```python
from build123d import *

# Parameters (mm, degrees)
F0_W     = 66.9
F0_H     = 51.6
F1_DEPTH = 1.5
F2_R     = 33.44999
F3_R     = 1.625
F4_DEPTH = 1.5
F5_W     = 5.2
F5_H     = 3.85
F5_W_2   = 5.05
F6_DEPTH = 1.7


# Not quite as in the source:
# - a fillet or chamfer is up to 0.001 mm smaller than in the source, because OpenCascade refuses the exact size


with BuildPart() as f1:
    # F0 (on Top) → F1 (new body)
    with BuildSketch(Plane.XY):
        Rectangle(F0_W, F0_H)
    extrude(amount=F1_DEPTH)

    # F2 (radius 33.45 in the source; OpenCascade refuses exactly that, so slightly less here)
    f2_edges = [f1.edges().sort_by_distance(p)[0] for p in [
        (-33.45, 25.8, 0.75),
        (33.45, 25.8, 0.75),
    ]]
    fillet(f2_edges, radius=F2_R)

    # F3 (on Top) → F4 (cut)
    with BuildSketch(Plane.XY):
        with Locations((-21.525, 14.0641658831)):
            Circle(F3_R)
        with Locations((-14.025, 12.9547324661)):
            Circle(F3_R)
        with Locations((21.525, 14.0641658831)):
            Circle(F3_R)
        with Locations((14.025, 12.9547324661)):
            Circle(F3_R)
        with Locations((-29.5, -14.475)):
            Circle(F3_R)
        with Locations((29.5, -14.475)):
            Circle(F3_R)
    extrude(amount=F4_DEPTH, mode=Mode.SUBTRACT)

    # F5 (on face) → F6 (join)
    with BuildSketch(Plane.XY.offset(1.5)):
        with Locations((0, -7.525)):
            Rectangle(F5_W, F5_H)
        with Locations((0.075, 12.975)):
            Rectangle(F5_W_2, F5_H)
    extrude(amount=F6_DEPTH)


solid = f1.part
```
Verification items for the finished model (mm, model axes). A direction names the side the tool comes from. Coordinates: 2 decimals unless noted, no trailing zeros. Write each loop counter-clockwise with the first axis right and the second up, starting at its lowest first coordinate (ties: lowest second). Pieces come first, ordered by that corner, then holes. Notation, with made-up numbers: (62.5, 29) - (117.5, 29) arc R18 ccw to (117.5, 37) - close; hole circle Ø2 at (-24, 31.5). An arc over 180 degrees is marked (long way). Write item = value, one per line.
Q1. Access from +Z, -Z, +X, -X, +Y, -Y to the whole of each face (thin tool, end or side, straight path). Record for faces 1 (the face through (0, -5.6, 2)), 2 (the face through (-2.45, 13, 2)), 3 (the face through (2.6, -8, 2)), 4 (the face through (21.17, 12.48, 0.74)), 5 (the face through (0, 14.9, 2)).
Answer:
face_1 = +Z, +X, -X
face_2 = +Z, -X, +Y
face_3 = +Z, +X, +Y, -Y
face_4 = +Z, -Z
face_5 = +Z, +X, -X, +Y
Q2. Cross-section at C-C (x = -17.5). Enter the section's corners in (y, z).
Answer:
outline = (-25.8, 0) - (20.86, 0) - (20.86, 1.5) - (-25.8, 1.5) - close
Q3. Cross-section at A-A (z = 2.25). Enter the section's corners in (x, y), plus the area to 3 significant figures.
Answer:
outline = (-2.6, -9.45) - (2.6, -9.45) - (2.6, -5.6) - (-2.6, -5.6) - close; (-2.45, 11.05) - (2.6, 11.05) - (2.6, 14.9) - (-2.45, 14.9) - close
area = 39.5 mm²
Q4. Material ranges on L1, parallel to Y at x = 0, z = 1.85; L2, parallel to X at y = 11.5, z = 1.85; L3, parallel to Z at x = -13.5, y = -4, recorded low to high. Write a range as from..to.
Answer:
L1 = -9.45..-5.6, 11.05..14.9
L2 = -2.45..2.6
L3 = 0..1.5
Q5. Cross-section at B-B (x = -29.5). Enter the section's corners in (y, z), plus the area to 3 significant figures.
Answer:
outline = (-25.8, 0) - (-16.1, 0) - (-16.1, 1.5) - (-25.8, 1.5) - close; (-12.85, 0) - (8.12, 0) - (8.12, 1.5) - (-12.85, 1.5) - close
area = 46.0 mm²
Q6. Mould release check, pull along Z, two halves, no side actions. Record for faces 6 (the face through (12.735, 11.966, 0.74)), 7 (the face through (0, -5, 0)), 8 (the face through (0, -7, 3.2)): released by +Z, released by -Z, zero draft, split by the parting line, or undercut.
Answer:
face_6 = zero draft
face_7 = released by -Z
face_8 = released by +Z
Q7. Go/stop test with flat-tipped pins: pin 1 Ø3.5 at (x, y) = (14.02, 12.95) entering from +Z; pin 2 Ø2.5 at (x, y) = (-21.52, 14.06) entering from -Z; pin 3 Ø1.9 at (x, z) = (1, 2.5) entering from -Y; pin 4 Ø1.9 at (y, z) = (-6.5, 2) entering from -X. Record where each tip stops, or that it passes through.
Answer:
pin_1 = 1.5
pin_2 = through
pin_3 = -9.45
pin_4 = -33.45
Q8. Cross-section at D-D (x = 24.5). Enter the section's corners in (y, z), plus the area to 3 significant figures.
Answer:
outline = (-25.8, 0) - (15.12, 0) - (15.12, 1.5) - (-25.8, 1.5) - close
area = 61.4 mm²
